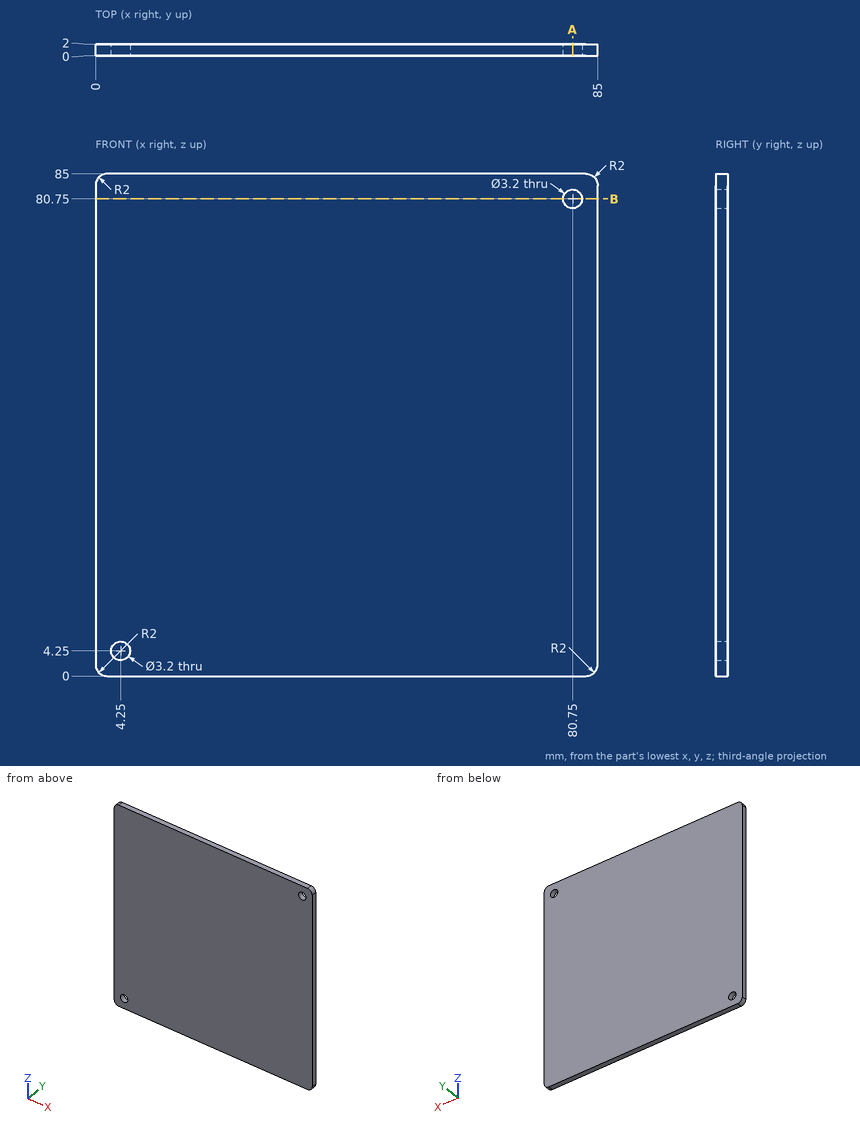
Source: three-view drawing plus pictorial views. Frame: mm from the lowest corner of the part. Give positions to 0.01 mm unless a question says otherwise; leave off trailing zeros. Order: outer loops, then holes, each group sorted by start corner. A loop starts at its lowest first (then second) coordinate and runs counter-clockwise, first axis right, second up. Notation, with made-up numbers: M 60.5,-7.5 L 119.5,-7.5 A24 ccw 119.5,29.5 Z; hole C 27,48 d4. An arc over 180 degrees is marked long. One line per question, with ' | ' between items.
1) Section A-A on x = 80.75. Output: boundary loops of the cut face in (y, z), and give its area (3 significant figures).
Filled in:
outline: M 0,0 L 2,0 L 2,79.15 L 0,79.15 Z; M 0,82.35 L 2,82.35 L 2,85 L 0,85 Z | area: 164 mm2
2) Section B-B on z = 80.75. Output: boundary loops of the cut face in (x, y).
Filled in:
outline: M 0,0 L 79.15,0 L 79.15,2 L 0,2 Z; M 82.35,0 L 85,0 L 85,2 L 82.35,2 Z
3) Ray query, L1, parallel to X at y = 0.5, z = 4.25; L2, parallel to X at y = 1.3, z = 80.75. Return the intervals inside material, ascending.
Filled in:
L1: x = 0 to 2.65, 5.85 to 85 | L2: x = 0 to 79.15, 82.35 to 85
